```python
from build123d import *

# Parameters (mm, degrees)
F0_W      = 125
F0_H      = 7
F1_DEPTH  = 105
F2_W      = 75
F2_H      = 60
F3_DEPTH  = 10
F4_W      = 75
F4_H      = 60
F5_DEPTH  = 10
F7_DEPTH  = 30
F8_R      = 30
F9_DEPTH  = 10
F10_R     = 17.5
F11_DEPTH = 5
F12_R     = 10
F13_DEPTH = 5


with BuildPart() as f1:
    # F0 (on Front) → F1 (new body)
    with BuildSketch(Plane.XZ):
        with Locations((1.324901, -12.605666)):
            Rectangle(F0_W, F0_H)
    extrude(amount=F1_DEPTH)

    # F2 (on face) → F3 (join)
    with BuildSketch(Plane.XZ.offset(105)):
        Polygon((-61.175099, -9.105666), (-61.175099, -16.105666), (63.824901, -16.105666), (63.824901, -9.105666), (38.824901, -9.105666), (-36.175099, -9.105666), align=None)
        with Locations((1.324901, 20.894334)):
            Rectangle(F2_W, F2_H)
        with BuildLine():
            ThreePointArc((38.824901, 50.894334), (1.324901, 88.394334), (-36.175099, 50.894334))
            Line((-36.175099, 50.894334), (38.824901, 50.894334))
        make_face()
    extrude(amount=F3_DEPTH)

    # F4 (on face) → F5 (join)
    with BuildSketch(Plane(origin=(0, 0, 0), x_dir=(-1, 0, 0), z_dir=(0, 1, 0))):
        Polygon((-63.824901, -9.105666), (-63.824901, -16.105666), (61.175099, -16.105666), (61.175099, -9.105666), (36.175099, -9.105666), (-38.824901, -9.105666), align=None)
        with Locations((-1.324901, 20.894334)):
            Rectangle(F4_W, F4_H)
        with BuildLine():
            ThreePointArc((36.175099, 50.894334), (-1.324901, 88.394334), (-38.824901, 50.894334))
            Line((-38.824901, 50.894334), (36.175099, 50.894334))
        make_face()
    extrude(amount=F5_DEPTH)

    # F6 (on face) → F7 (join)
    with BuildSketch(Plane(origin=(0, 0, -16.105666), x_dir=(1, 0, 0), z_dir=(0, 0, -1))):
        with BuildLine():
            ThreePointArc((18.824901, 52.5), (13.699269, 64.874369), (1.324901, 70))
            Line((1.324901, 70), (1.324901, 52.5))
            Line((1.324901, 52.5), (18.824901, 52.5))
        make_face()
        with BuildLine():
            Line((1.324901, 52.5), (1.324901, 70))
            ThreePointArc((1.324901, 70), (-11.049468, 64.874369), (-16.175099, 52.5))
            Line((-16.175099, 52.5), (1.324901, 52.5))
        make_face()
        with BuildLine():
            Line((18.824901, 52.5), (1.324901, 52.5))
            Line((1.324901, 52.5), (1.324901, 35))
            ThreePointArc((1.324901, 35), (13.699269, 40.125631), (18.824901, 52.5))
        make_face()
        with BuildLine():
            Line((1.324901, 35), (1.324901, 52.5))
            Line((1.324901, 52.5), (-16.175099, 52.5))
            ThreePointArc((-16.175099, 52.5), (-11.049468, 40.125631), (1.324901, 35))
        make_face()
    extrude(amount=F7_DEPTH)

    # F8 (on face) → F9 (join)
    with BuildSketch(Plane(origin=(0, 0, -46.105666), x_dir=(1, 0, 0), z_dir=(0, 0, -1))):
        with Locations((1.324901, 52.5)):
            Circle(F8_R)
    extrude(amount=F9_DEPTH)

    # F10 (on face) → F11 (cut)
    with BuildSketch(Plane(origin=(0, 0, -56.105666), x_dir=(1, 0, 0), z_dir=(0, 0, -1))):
        with Locations((1.324901, 52.5)):
            Circle(F10_R)
    extrude(amount=-F11_DEPTH, mode=Mode.SUBTRACT)

    # F12 (on face) → F13 (cut)
    with BuildSketch(Plane(origin=(0, 0, -51.105666), x_dir=(1, 0, 0), z_dir=(0, 0, -1))):
        with Locations((1.324901, 52.5)):
            Circle(F12_R)
    extrude(amount=-F13_DEPTH, mode=Mode.SUBTRACT)


solid = f1.part
```
Source: CAD feature listing. Evaluate the final solid. Frame: model axes, mm. A direction names the side the tool comes from. Coordinates: 2 decimals unless noted, no trailing zeros. Loops run counter-clockwise (first coordinate to the right, second up) from the corner with the lowest first, then second, coordinate; pieces in that order, holes last. Notation, with made-up numbers: (64.25, 49) -> (105.25, 49) arc R18 cw to (105.25, 63) -> close; hole circle Ø10 at (73.5, -34). An arc over 180 degrees is marked (long way). One line per item, written item: value. Start each with the question number.
Q1. Section query B-B, the plane y = -26. Return the cut outline in (x, z).
Q2. Mould query, pull axis X, two halves, no side actions, for faces 1 (the face through (-5.179, -23.213, -51.036)), 2 (the face through (0, -53, -9.106)), 3 (the face through (-0.843, -42.738, -48.641)), 4 (the face through (-2.469, -35.416, -53.641)). Classes: pulls with the +X half, pulls with the -X half, needs draft (parallel to the pull), parting line crosses it, or undercut.
Q3. Set-up query: faces 5 (the face through (-36.175, 5, 20)), 6 (the face through (1, -105, 40)), 7 (the face through (38.825, 5, 20)). Return all of +Z, -Z, +X, -X, +Y, -Y with unobstructed straight access to the full face (end or side cutting, diameter ignored); none if empty.
Q4. Line query: line 1 along Y through (x, z) = (-8, 31.5); line 2 along X through (y, z) = (-52, -48); line 3 along Z through (x, y) = (-2.5, -30). Output: solid intervals per line, ascending.
Q5. Section query D-D, the plane y = -58.5. Return the cut outline in (x, z).
Q6. Section query C-C, the plane x = -25.5. Return the cut outline in (y, z), and give its area (3 significant figures).
Q7. Section query A-A, the plane z = 49. Return the cut outline in (x, y), and give its area (3 significant figures).
Q8. Contact query for flat-ended pins moving along their axis: P1, Ø10, axis at x = -1, y = -50, coming from the -Z side; P2, Ø2, axis at x = 42.5, y = -68, coming from the -Z side; P3, Ø3, axis at y = -108, z = 14.5, coming from the -X side; P4, Ø10, axis at x = 48.5, z = -8.5, coming from the -Y side. Output: stop coordinate, or through.
Results:
1. outline: (-61.18, -16.11) -> (63.82, -16.11) -> (63.82, -9.11) -> (-61.18, -9.11) -> close; (-12.74, -56.11) -> (15.39, -56.11) -> (15.39, -46.11) -> (-12.74, -46.11) -> close
2. face 1: parting line crosses it
2. face 2: needs draft
2. face 3: undercut
2. face 4: undercut
3. face 5: +Z, -X, +Y, -Y
3. face 6: +Z, +X, -X
3. face 7: +Z, +X, +Y, -Y
4. line 1: -115 to -105, 0 to 10
4. line 2: -28.67 to -8.66, 11.31 to 31.32
4. line 3: -56.11 to -46.11, -16.11 to -9.11
5. outline: (-61.18, -16.11) -> (-15.11, -16.11) -> (-15.11, -46.11) -> (-28.07, -46.11) -> (-28.07, -56.11) -> (-15.11, -56.11) -> (-15.11, -51.11) -> (-6.68, -51.11) -> (-6.68, -46.11) -> (9.32, -46.11) -> (9.32, -51.11) -> (17.76, -51.11) -> (17.76, -56.11) -> (30.72, -56.11) -> (30.72, -46.11) -> (17.76, -46.11) -> (17.76, -16.11) -> (63.82, -16.11) -> (63.82, -9.11) -> (-61.18, -9.11) -> close
6. outline: (-115, -16.11) -> (10, -16.11) -> (10, 77.1) -> (0, 77.1) -> (0, -9.11) -> (-105, -9.11) -> (-105, 77.1) -> (-115, 77.1) -> close; (-65.93, -56.11) -> (-39.07, -56.11) -> (-39.07, -46.11) -> (-65.93, -46.11) -> close
6. area: 2,870 mm^2
7. outline: (-36.18, -115) -> (38.82, -115) -> (38.82, -105) -> (-36.18, -105) -> close; (-36.18, 0) -> (38.82, 0) -> (38.82, 10) -> (-36.18, 10) -> close
7. area: 1,500 mm^2
8. P1: z = -46.11
8. P2: z = -16.11
8. P3: x = -36.18
8. P4: y = -115
